Autodesk Inventor part; units mm, degrees
ref_plane "YZ Plane" through (0, 0, 0) normal (1, 0, 0) x (0, 1, 0)
ref_plane "XZ Plane" through (0, 0, 0) normal (0, 1, 0) x (-1, 0, 0)
ref_plane "XY Plane" through (0, 0, 0) normal (0, 0, 1) x (1, 0, 0)
sketch "Sketch1" plane through (0, 0, 0) normal (0, 0, 1) x (1, 0, 0)
  line L0 (15.7385, -0.0311) -> (-29.1749, -0.0311)
  line L1 (-29.1749, -0.0311) -> (2.0558, -0.0311) construction
  line L2 (-29.1749, -8.0311) -> (-19.1749, -8.0311)
  line L3 (-19.1749, -8.0311) -> (-9.0765, -8.6728) construction
  line L4 (-9.0765, -8.6728) -> (-1.6699, -24.4547) construction
  spline S0 degree 2 poles (-19.1749, -8.0311) (-9.0765, -8.6728) (-1.6699, -24.4547) knots 1 1 1 2 2 2
  line L5 (-1.6699, -24.4547) -> (2.9761, -22.4111) construction
  line L6 (2.9761, -22.4111) -> (-2.9231, -11.7108) construction
  spline S1 degree 2 poles (-1.6699, -24.4547) (2.9761, -22.4111) (-2.9231, -11.7108) knots 1 1 1 2 2 2
  line L7 (-2.9231, -11.7108) -> (-2.9231, -4.7242) construction
  line L8 (-2.9231, -4.7242) -> (18.0519, -6.1311) construction
  line L9 (18.0519, -6.1311) -> (15.7385, -0.0311) construction
  spline S2 degree 3 poles (-2.9231, -11.7108) (-2.9231, -4.7242) (18.0519, -6.1311) (15.7385, -0.0311) knots 1 1 1 1 2 2 2 2
  arc A0 (-29.1749, -0.0311) -> (-29.1749, -8.0311) centre (-29.1749, -4.0311) ccw
  circle A1 centre (-29.1749, -4.0311) radius 2.25
  point P0 (0, 0)
  dimension "d0" = 8
  dimension "d1" = 10
  dimension "d2" = 4.5
extrude "Extrusion1" add sketch "Sketch1" along normal blind 3
sketch "Sketch2" plane through (0, 0, 3) normal (0, 0, 1) x (1, 0, 0)
  line L0 (15.7385, -0.0311) -> (-29.1749, -0.0311)
  line L1 (-29.1749, -0.0311) -> (-1.8249, -0.0311)
  circle A0 centre (-1.8249, -0.0311) radius 3.5
  point P0 (0, 0)
  dimension "d5" = 27.35
  dimension "d6" = 7
extrude "Extrusion2" cut sketch "Sketch2" against normal blind 3
sketch "Sketch3" plane through (0, 0, 3) normal (0, 0, 1) x (1, 0, 0)
  line L0 (-1.6699, -24.4547) -> (-2.4199, -23.1557)
  line L1 (-1.6699, -24.4547) -> (-0.1699, -24.4547) construction
  line L2 (-3.7341, -20.8795) -> (-2.4199, -23.1557)
  line L3 (-2.4199, -23.1557) -> (-1.13, -22.0176) construction
  line L4 (-1.13, -22.0176) -> (-2.0449, -20.2761) construction
  line L5 (-2.0449, -20.2761) -> (-3.7341, -20.8795) construction
  spline S0 degree 3 poles (-2.4199, -23.1557) (-1.13, -22.0176) (-2.0449, -20.2761) (-3.7341, -20.8795) knots 1 1 1 1 2 2 2 2
  point P0 (0, 0)
  dimension "d9" = 1.5
  dimension "d10" = 120
extrude "Extrusion3" cut sketch "Sketch3" against normal blind 3
fillet "Fillet2" radius 2 1 edges at (-3.5248, -20.8155, 1.5)
chamfer "Chamfer1" distance 1.2 angle 45 1 edges at (-31.4249, -4.0311, 0)
fillet "Fillet4" radius 1 2 edges at (1.6751, -0.0311, 1.5) (-5.3249, -0.0311, 1.5)
properties part number "retreat"
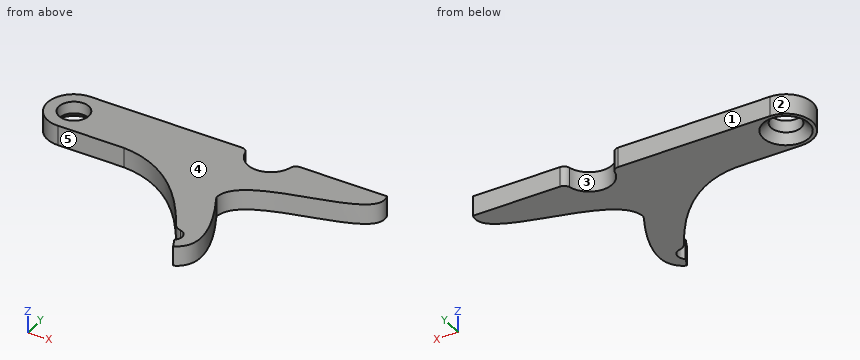
CAD build for the part. Positions are in the model's coordinates, mm. Face numbers are marked on the shaded views. A direction names the side the tool comes from. Coordinates: 2 decimals unless noted, no trailing zeros. Write each loop counter-clockwise with the first axis right and the second up, starting at its lowest first coordinate (ties: lowest second). Pieces come first, ordered by that corner, then holes.
(1) Drill centre lines: probe 1 along Y at (x, z) = (-2, 2.45); probe 2 along Y at (x, z) = (-30, 1.4); probe 3 along Y at (x, z) = (-29.5, 0.65). Where is each one in solid material? Low to high.
(2) Flat gauge pin, fed straight in: pin 1 (5 mm diameter, centred on x = -29.17, y = -4.03, fed in from +Z). Where does the tip first touch, or does it go through?
(3) Two-plate mould, pull along X, no slides. Class the marked faces 1, 2 and 3: +X half, -X half, draft (parallel to the pull), parting line (faces both ways), or undercut.
(4) Cut at A-A, the plane x = -21.5. List the corners of the cut face in (y, z), and give its area (3 significant figures).
(5) 3-axis set-ups, long thin cutter, end or side, ignore diameter. For the marked faces 4 and 5: which of +Z, -Z, +X, -X, +Y, -Y reach the whole face in a straight line?
Geometry says:
1. probe 1: y = -23.76 to -22.64, -21.3 to -13.46, -9.42 to -3.53
1. probe 2: y = -7.95 to -6.12, -1.94 to -0.12
1. probe 3: y = -8.02 to -6.81, -1.25 to -0.04
2. pin 1: stops at z = 3
3. face 1: draft
3. face 2: -X half
3. face 3: undercut
4. outline: (-8.03, 0) - (-0.03, 0) - (-0.03, 3) - (-8.03, 3) - close
4. area: 24.0 mm2
5. face 4: +Z, +X, -X, +Y, -Y
5. face 5: +Z, -Z, -X, -Y
